from build123d import *
from OCP.BRepFilletAPI import BRepFilletAPI_MakeChamfer

# Parameters (mm, degrees)
BOSS_EXTRUDE1_DEPTH     = 6.5
SKETCH2_R               = 1.575
CUT_EXTRUDE1_DEPTH      = 75.74790967
CUT_EXTRUDE2_START      = 5
SKETCH2_3_R             = 3
CUT_EXTRUDE2_DEPTH      = 70.74790967
CUT_EXTRUDE3_DEPTH      = 75.74790967
CUT_EXTRUDE3_DEPTH_BACK = 75.74790967
CHAMFER1_SIZE           = 2
CHAMFER1_SIZE2          = 4.284869987
CHAMFER1_SIZE2_2        = 2.26145916
FILLET2_R               = 4


with BuildPart() as part:
    # Sketch1 → Boss-Extrude1 (new, symmetric)
    with BuildSketch(Plane(origin=(0, 0, 0), x_dir=(0, 0, -1), z_dir=(1, 0, 0))):
        Polygon((0, 19), (0, -19), (-72, -19), align=None)
    extrude(amount=BOSS_EXTRUDE1_DEPTH, both=True)

    # Sketch2 → Cut-Extrude1 (cut, through all)
    with BuildSketch(Plane.XY):
        with Locations(Location((0, 10.5, 0), (0, 0, 90))):
            Circle(SKETCH2_R)
        with Locations(Location((0, -10.5, 0), (0, 0, 180))):
            Circle(SKETCH2_R)
    extrude(amount=CUT_EXTRUDE1_DEPTH, mode=Mode.SUBTRACT)

    # Sketch2_3 → Cut-Extrude2 (cut, through all)
    with BuildSketch(Plane.XY.offset(CUT_EXTRUDE2_START)):
        with Locations(Location((0, 10.5, 0), (0, 0, 90))):
            Circle(SKETCH2_3_R)
        with Locations(Location((0, -10.5, 0), (0, 0, 180))):
            Circle(SKETCH2_3_R)
    extrude(amount=CUT_EXTRUDE2_DEPTH, mode=Mode.SUBTRACT)

    # Sketch5 → Cut-Extrude3 (cut, two sides: drawn at the far end of the back side and taken through both)
    with BuildSketch(Plane(origin=(0, 0, 0), x_dir=(0, 0, -1), z_dir=(1, 0, 0)).offset(-CUT_EXTRUDE3_DEPTH_BACK)):
        with BuildLine():
            Line((-13.25, 1.25), (-10.75, 1.25))
            ThreePointArc((-10.75, 1.25), (-9.5, 0), (-10.75, -1.25))
            Line((-10.75, -1.25), (-13.25, -1.25))
            ThreePointArc((-13.25, -1.25), (-14.5, 0), (-13.25, 1.25))
        make_face()
    extrude(amount=CUT_EXTRUDE3_DEPTH + CUT_EXTRUDE3_DEPTH_BACK, mode=Mode.SUBTRACT)

    # Chamfer1: one chamfer whose edges measure the first distance from different faces: ONE call of the kernel's chamfer builder (chamfer() names one face for all edges)
    chamfer1_edges_1 = [part.edges().sort_by_distance(p)[0] for p in [
        (0, 19, 0),
    ]]
    chamfer1_side_1 = [part.faces().sort_by_distance(p)[0] for p in [
        (0, 0, 0),
    ]]
    chamfer1_edges_2 = [part.edges().sort_by_distance(p)[0] for p in [
        (0, -19, 72),
    ]]
    chamfer1_side_2 = [part.faces().sort_by_distance(p)[0] for p in [
        (0, -19, 36),
    ]]
    chamfer1 = BRepFilletAPI_MakeChamfer(part.part.solid().wrapped)
    for e in chamfer1_edges_1:
        chamfer1.Add(CHAMFER1_SIZE, CHAMFER1_SIZE2, e.wrapped, chamfer1_side_1[0].wrapped)  # the first distance lies on this face
    for e in chamfer1_edges_2:
        chamfer1.Add(CHAMFER1_SIZE, CHAMFER1_SIZE2_2, e.wrapped, chamfer1_side_2[0].wrapped)  # the first distance lies on this face
    add(Compound.cast(chamfer1.Shape()), mode=Mode.REPLACE)

    # Fillet2
    fillet2_edges = [part.edges().sort_by_distance(p)[0] for p in [
        (-6.5, 17, 1.894736842),
        (-6.5, -18.472222222, 70),
        (6.5, 17, 1.894736842),
        (6.5, -18.472222222, 70),
    ]]
    fillet(fillet2_edges, radius=FILLET2_R)


solid = part.part
Geometry: final body of the model. Coordinates: model frame, mm. A direction names the side the tool comes from. Give positions to 0.01 mm unless a question says otherwise; leave off trailing zeros. Write each loop counter-clockwise with the first axis right and the second up, starting at its lowest first coordinate (ties: lowest second). Pieces come first, ordered by that corner, then holes. Notation, with made-up numbers: (5, 40) - (14, 40) arc R21 ccw to (14, 48) - close; hole circle Ø11 at (-38.5, 65). An arc over 180 degrees is marked (long way). Return JSON: item names as keys, results as strings. Group by question number.
1) Section D-D on y = 10.5. Return the cut outline in (x, z) (3 decimals).
2) Section B-B on x = -5. Return the cut outline in (y, z), plus the area to 3 significant figures.
3) Line query: line 1 (Y direction, x = 0, z = 11.5); line 2 (X direction, y = -10.5, z = 6); line 3 (Y direction, x = 0.25, z = 16). Output: solid intervals per line, ascending.
4) First-contact query: P1, Ø5, axis at x = 1.5, y = -12, coming from the +Z side; P2, Ø1.8, axis at x = -1.5, y = -11, coming from the +Z side; P3, Ø0.8, axis at x = 0, z = 12.5, coming from the +Y side. Flat tips, straight axial feed; report the tip coordinate or a pass-through.
5) Set-up query: faces 1 (the cylindrical face through (-0.1, 7.5, 11.5)), 2 (the flat face through (0, 1.25, 12)), 3 (the cylindrical face through (-5.8, -18.1, 68.26)). Return all of +Z, -Z, +X, -X, +Y, -Y with unobstructed straight access to the full face (end or side cutting, diameter ignored); none if empty.
6) Mould query, pull axis Y, two halves, no side actions, for faces 4 (the cylindrical face through (-5.8, 15.26, 3.24)), 5 (the flat face through (0, -1, 0)), 6 (the cylindrical face through (0.391, -13.474, 32.96)). Classes: released by +Y, released by -Y, zero draft, split by the parting line, or undercut.
7) Section C-C on z = 52.5. Return the cut outline in (x, y), plus the area to 3 significant figures.
8) Section A-A on y = 0. Return the cut outline in (x, z).
Filled in:
{
 "1": {"outline": "(-6.5, 0) - (-1.575, 0) - (-1.575, 5) - (-3, 5) - (-3, 16.105) - (-6.5, 16.105) - close; (1.575, 0) - (6.5, 0) - (6.5, 16.105) - (3, 16.105) - (3, 5) - (1.575, 5) - close"},
 "2": {"outline": "(-19, 0) - (16.12, 0) - (16.12, 5.45) - (-17.48, 69.12) - (-19, 69.12) - close; hole (-1.25, 10.75) arc R1.25 ccw to (1.25, 10.75) - (1.25, 13.25) arc R1.25 ccw to (-1.25, 13.25) - close", "area": "1,350 mm^2"},
 "3": {"line 1": "y = -19 to -13.5, -7.5 to -1.25, 1.25 to 7.5", "line 2": "x = -6.5 to -3, 3 to 6.5", "line 3": "y = -19 to -13.49, -7.51 to 7.51"},
 "4": {"P1": "stops at z = 63.47", "P2": "stops at z = 5", "P3": "stops at y = 7.53"},
 "5": {"face 1": "+Z", "face 2": "+X, -X", "face 3": "+Z, -X, +Y, -Y"},
 "6": {"face 4": "released by +Y", "face 5": "zero draft", "face 6": "undercut"},
 "7": {"outline": "(-6.5, -19) - (6.5, -19) - (6.5, -8.71) - (2.41, -8.71) arc R3 cw (long way) to (-2.41, -8.71) - (-6.5, -8.71) - close", "area": "110 mm^2"},
 "8": {"outline": "(-6.5, 0) - (6.5, 0) - (6.5, 9.5) - (-6.5, 9.5) - close; (-6.5, 14.5) - (6.5, 14.5) - (6.5, 36) - (-6.5, 36) - close"}
}
